Autodesk Inventor part; units mm, degrees
ref_plane "YZ Plane" through (0, 0, 0) normal (1, 0, 0) x (0, 1, 0)
ref_plane "XZ Plane" through (0, 0, 0) normal (0, 1, 0) x (-1, 0, 0)
ref_plane "XY Plane" through (0, 0, 0) normal (0, 0, 1) x (1, 0, 0)
sketch "Sketch1" plane through (0, 0, 0) normal (0, 1, 0) x (-1, 0, 0)
  line L0 (0, 0) -> (25.4, 0)
  line L1 (25.4, 0) -> (25.4, 50.8)
  line L2 (25.4, 50.8) -> (0, 50.8)
  line L3 (0, 50.8) -> (0, 0)
  dimension "d0" = 50.8
  dimension "d1" = 25.4
extrude "Extrusion1" add sketch "Sketch1" along normal blind 1295.4
sketch "Sketch2" plane through (0, 0, 50.8) normal (0, 0, 1) x (1, 0, 0)
  line L0 (-9.525, 0) -> (-15.875, 0)
  line L1 (-15.875, 0) -> (-15.875, 1295.4)
  line L2 (-25.4, 0) -> (-25.4, 1295.4)
  line L3 (0, 1295.4) -> (-25.4, 1295.4)
  line L4 (-9.525, 1295.4) -> (-9.525, 0)
  line L5 (0, 0) -> (0, 1295.4)
  line L6 (0, 0) -> (-25.4, 0)
  line L7 (-15.875, 1295.4) -> (-9.525, 1295.4)
  dimension "d4" = 9.525
  dimension "d5" = 6.35
  dimension "d6" = 9.525
  dimension "d9" = 9.525
extrude "Extrusion2" cut sketch "Sketch2" against normal blind 8.4667 contours L0 L1 L3 L4
sketch "Sketch3" plane through (-25.4, 0, 0) normal (0, 0, -1) x (-1, 0, 0)
  line L0 (-15.875, 0) -> (-9.525, 0)
  line L1 (-9.525, 0) -> (-9.525, 1295.4)
  line L2 (-9.525, 1295.4) -> (-15.875, 1295.4)
  line L3 (-15.875, 1295.4) -> (-15.875, 0)
  point P0 (-25.4, 0)
extrude "Extrusion3" cut sketch "Sketch3" against normal blind 8.4667
sketch "Sketch4" plane through (-25.4, 0, 0) normal (-1, 0, 0) x (0, 0, 1)
  line L0 (0, 1295.4) -> (50.8, 1295.4)
  line L1 (9.525, 0) -> (15.875, 0)
  line L2 (15.875, 0) -> (15.875, 1295.4)
  line L3 (15.875, 1295.4) -> (9.525, 1295.4)
  line L4 (9.525, 1295.4) -> (9.525, 0)
  line L5 (35.9833, 1295.4) -> (42.3333, 1295.4)
  line L6 (42.3333, 1295.4) -> (42.3333, 0)
  line L7 (42.3333, 0) -> (35.9833, 0)
  line L8 (35.9833, 0) -> (35.9833, 1295.4)
  line L9 (0, 0) -> (0, 1295.4)
  point P0 (50.8, 0)
  dimension "d14" = 9.525
  dimension "d16" = 6.35
  dimension "d17" = 6.35
  dimension "d18" = 9.525
extrude "Extrusion4" cut sketch "Sketch4" against normal blind 8.4667
sketch "Sketch5" plane through (0, 0, 50.8) normal (1, 0, 0) x (0, 0, -1)
  line L0 (8.4667, 0) -> (14.8167, 0)
  line L1 (14.8167, 0) -> (14.8167, 1295.4)
  line L2 (14.8167, 1295.4) -> (8.4667, 1295.4)
  line L3 (8.4667, 1295.4) -> (8.4667, 0)
  line L4 (34.925, 1295.4) -> (41.275, 1295.4)
  line L5 (41.275, 1295.4) -> (41.275, 0)
  line L6 (41.275, 0) -> (34.925, 0)
  line L7 (34.925, 0) -> (34.925, 1295.4)
  point P0 (50.8, 0)
extrude "Extrusion5" cut sketch "Sketch5" against normal blind 8.4667
properties part number "HammerStick Stick"
Work out the finished part from the listing and answer in its coordinate system (mm). Give positions to 0.01 mm unless a question says otherwise; leave off trailing zeros. Order: outer loops, then holes, each group sorted by start corner. A loop starts at its lowest first (then second) coordinate and runs counter-clockwise, first axis right, second up. Notation, with made-up numbers: (81, 68) - (110, 68) arc R21 ccw to (110, 101) - close; hole circle Ø4 at (-26.5, -29.5). An arc over 180 degrees is marked (long way). One line per item, written item: value. Start each with the question number.
1. Consider line 1 (Z direction, x = -17.75, y = 1149) (3 decimals); line 2 (X direction, y = 920.5, z = 8) (3 decimals); line 3 (Z direction, x = -14.75, y = 347.5). Determine where each line is inside the solid, lowest interval first.
2. This flat-tipped pin is pushed along its axis until it touches: pin 1 Ø1.9 at (y, z) = (440, 38) entering from -X. Where does it stop, or does it pass through?
3. Section B-B, the plane y = 1091 is taken. Write down the section's boundary in (x, z) (3 decimals).
4. Section A-A, the plane x = -21.5 is taken. Write down the section's boundary in (y, z) (3 decimals), then the cut area to 3 significant figures.
Filled sheet:
1. line 1: 0 to 9.525, 15.875 to 35.983, 42.333 to 50.8
1. line 2: -25.4 to -15.875, -9.525 to 0
1. line 3: 8.47 to 42.33
2. pin 1: x = -16.93
3. outline: (-25.4, 0) - (-15.875, 0) - (-15.875, 8.467) - (-9.525, 8.467) - (-9.525, 0) - (0, 0) - (0, 9.525) - (-8.467, 9.525) - (-8.467, 15.875) - (0, 15.875) - (0, 35.983) - (-8.467, 35.983) - (-8.467, 42.333) - (0, 42.333) - (0, 50.8) - (-9.525, 50.8) - (-9.525, 42.333) - (-15.875, 42.333) - (-15.875, 50.8) - (-25.4, 50.8) - (-25.4, 42.333) - (-16.933, 42.333) - (-16.933, 35.983) - (-25.4, 35.983) - (-25.4, 15.875) - (-16.933, 15.875) - (-16.933, 9.525) - (-25.4, 9.525) - close
4. outline: (0, 0) - (1295.4, 0) - (1295.4, 9.525) - (0, 9.525) - close; (0, 15.875) - (1295.4, 15.875) - (1295.4, 35.983) - (0, 35.983) - close; (0, 42.333) - (1295.4, 42.333) - (1295.4, 50.8) - (0, 50.8) - close
4. area: 49,400 mm²
